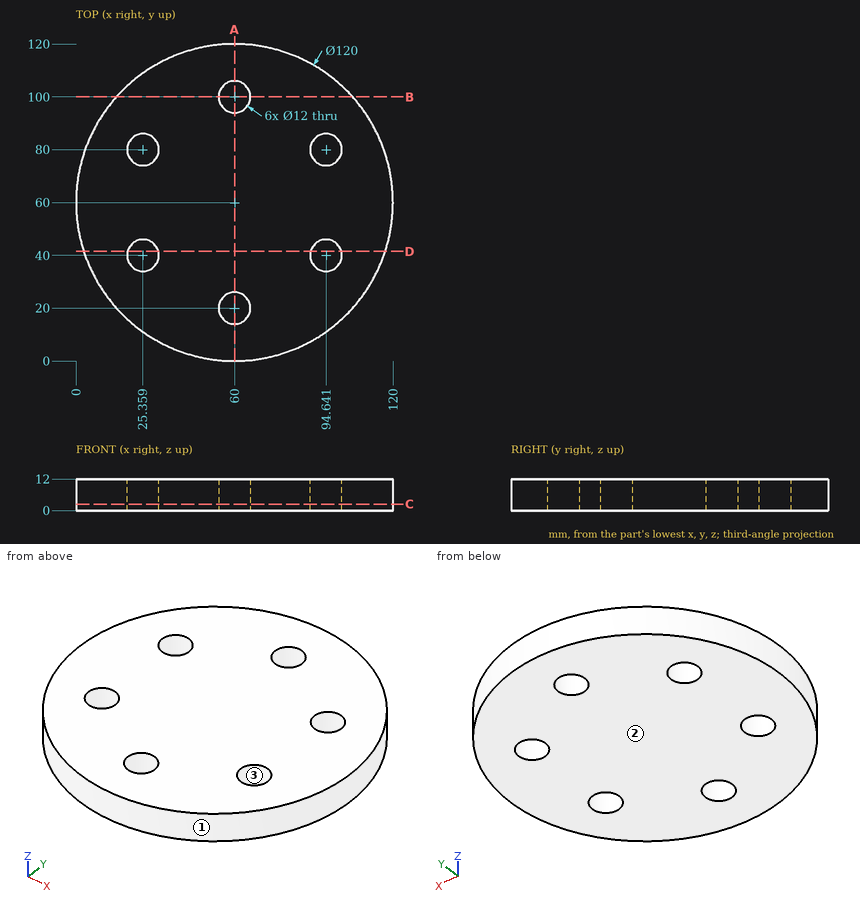
Could you check a few things on this drawing? It's one solid part, dimensions in mm from its lowest x, y, z. Round coordinates to 2 decimals unless told otherwise and drop trailing zeros. Loops run counter-clockwise (first coordinate to the right, second up) from the corner with the lowest first, then second, coordinate; pieces in that order, holes last. Notation, with made-up numbers: M 13.25,-2 L 34.25,-2 A23 cw 34.25,35 Z; hole C 5,29 d5. An arc over 180 degrees is marked long. Write each question's results on one line, items separated by ' | '. Start each with the question number.
(1) I want a section at A-A (x = 60). Please give me the cut outline in (y, z), then the cut area to 3 significant figures.
(2) I want a section at B-B (y = 100). Please give me the cut outline in (x, z), then the cut area to 3 significant figures.
(3) If I drill on probe 1 along Y at (x, z) = (60, 4.25); probe 2 along X at (y, z) = (39.5, 1.5); probe 3 along Y at (x, z) = (62, 5.5), over which ranges is the centre line in solid material (lowest first)? Write a range as from..to.
(4) I want a section at D-D (y = 41.5). Please give me the cut outline in (x, z).
(5) Thinking about a two-plate mould opening in Y: for the marked faces 1, 2 and 3, which applies, pulls with the +Y half, pulls with the -Y half, needs draft (parallel to the pull), parting line crosses it, or undercut?
(6) I want a section at C-C (z = 2.5). Please give me the cut outline in (x, y).
(7) Will these pins go through, and if not, where does the flat tip stop? P1, Ø19, axis at x = 94.64, y = 40, coming from the -Z side; P2, Ø2, axis at x = 56, z = 7, coming from the +Y side (3 decimals); P3, Ø4, axis at x = 91.5, z = 1.5, coming from the +Y side; P4, Ø2, axis at x = 36, z = 7, coming from the -Y side.
Solved:
1) outline: M 0,0 L 14,0 L 14,12 L 0,12 Z; M 26,0 L 94,0 L 94,12 L 26,12 Z; M 106,0 L 120,0 L 120,12 L 106,12 Z | area: 1,150 mm²
2) outline: M 15.28,0 L 54,0 L 54,12 L 15.28,12 Z; M 66,0 L 104.72,0 L 104.72,12 L 66,12 Z | area: 929 mm²
3) probe 1: y = 0..14, 26..94, 106..120 | probe 2: x = 3.61..19.38, 31.34..88.66, 100.62..116.39 | probe 3: y = 0.03..14.34, 25.66..94.34, 105.66..119.97
4) outline: M 2.92,0 L 19.55,0 L 19.55,12 L 2.92,12 Z; M 31.17,0 L 88.83,0 L 88.83,12 L 31.17,12 Z; M 100.45,0 L 117.08,0 L 117.08,12 L 100.45,12 Z
5) face 1: parting line crosses it | face 2: needs draft | face 3: undercut
6) outline: C 60,60 d120; hole C 25.36,40 d12; hole C 25.36,80 d12; hole C 60,20 d12; hole C 60,100 d12; hole C 94.64,40 d12; hole C 94.64,80 d12
7) P1: stops at z = 0 | P2: stops at y = 119.925 | P3: stops at y = 112.25 | P4: stops at y = 4.58
